Can you work these out from the model? Positions are in its coordinate system, mm. Face numbers are marked on the shaded views. A direction names the side the tool comes from. Round coordinates to 2 decimals unless told otherwise and drop trailing zeros. Loops run counter-clockwise (first coordinate to the right, second up) from the corner with the lowest first, then second, coordinate; pieces in that order, holes last. Notation, with made-up numbers: (67.25, 79) - (116.25, 79) arc R23 ccw to (116.25, 115) - close; hole circle Ø1 at (41, -30.5). An arc over 180 degrees is marked (long way). Answer as CSV lines item,"result".
```python
from build123d import *

# Parameters (mm, degrees)
SKETCH1_W           = 50
SKETCH1_H           = 40
BOSS_EXTRUDE1_DEPTH = 50
SKETCH2_W           = 44
SKETCH2_H           = 44
CUT_EXTRUDE1_DEPTH  = 50
SKETCH3_R           = 1.7
CUT_EXTRUDE3_DEPTH  = 78.691698398
SKETCH5_R           = 9
CUT_EXTRUDE4_DEPTH  = 2
SKETCH6_R           = 3
CUT_EXTRUDE5_DEPTH  = 79.841613378
SKETCH7_R           = 1.7
CUT_EXTRUDE6_DEPTH  = 78.691698398


with BuildPart() as part:
    # Sketch1 → Boss-Extrude1 (new body)
    with BuildSketch(Plane(origin=(0, 0, 0), x_dir=(1, 0, 0), z_dir=(0, 1, 0))):
        with Locations((25, 20)):
            Rectangle(SKETCH1_W, SKETCH1_H)
    extrude(amount=BOSS_EXTRUDE1_DEPTH)

    # Sketch2 → Cut-Extrude1 (cut)
    with BuildSketch(Plane.XY):
        with Locations((22, 28)):
            Rectangle(SKETCH2_W, SKETCH2_H)
    extrude(amount=-CUT_EXTRUDE1_DEPTH, mode=Mode.SUBTRACT)

    # Sketch3 → Cut-Extrude3 (cut, through all)
    with BuildSketch(Plane.ZY.offset(-44)):
        with Locations(Location((-30, 40, 0), (0, 0, 270))):
            Circle(SKETCH3_R)
        with Locations(Location((-10, 40, 0), (0, 0, 270))):
            Circle(SKETCH3_R)
        with Locations(Location((-10, 16, 0), (0, 0, 270))):
            Circle(SKETCH3_R)
        with Locations(Location((-30, 16, 0), (0, 0, 270))):
            Circle(SKETCH3_R)
    extrude(amount=-CUT_EXTRUDE3_DEPTH, mode=Mode.SUBTRACT)

    # Sketch5 → Cut-Extrude4 (cut)
    with BuildSketch(Plane(origin=(0, 6, 0), x_dir=(1, 0, 0), z_dir=(0, 1, 0))):
        with Locations(Location((23, 20, 0), (0, 0, 270))):
            Circle(SKETCH5_R)
    extrude(amount=-CUT_EXTRUDE4_DEPTH, mode=Mode.SUBTRACT)

    # Sketch6 → Cut-Extrude5 (cut, through all)
    with BuildSketch(Plane(origin=(0, 4, 0), x_dir=(1, 0, 0), z_dir=(0, 1, 0))):
        with Locations(Location((23, 20, 0), (0, 0, 270))):
            Circle(SKETCH6_R)
    extrude(amount=-CUT_EXTRUDE5_DEPTH, mode=Mode.SUBTRACT)

    # Sketch7 → Cut-Extrude6 (cut, through all)
    with BuildSketch(Plane(origin=(0, 6, 0), x_dir=(1, 0, 0), z_dir=(0, 1, 0))):
        with Locations(Location((12, 20, 0), (0, 0, 270))):
            Circle(SKETCH7_R)
        with Locations(Location((23, 31, 0), (0, 0, 270))):
            Circle(SKETCH7_R)
        with Locations(Location((34, 20, 0), (0, 0, 270))):
            Circle(SKETCH7_R)
        with Locations(Location((23, 9, 0), (0, 0, 270))):
            Circle(SKETCH7_R)
    extrude(amount=-CUT_EXTRUDE6_DEPTH, mode=Mode.SUBTRACT)


solid = part.part
```
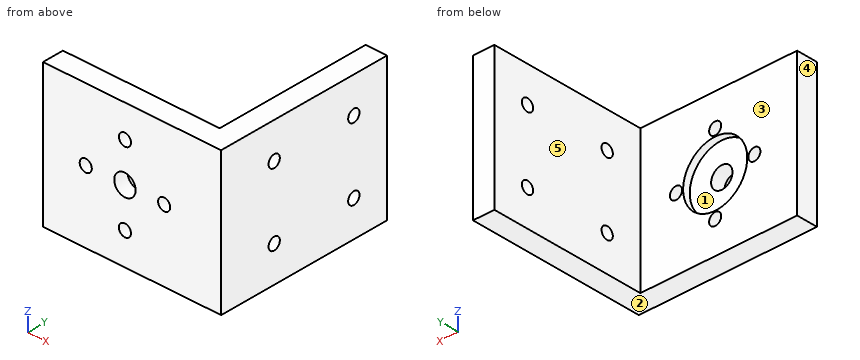
Q1. I'm going to push flat-ended pins straight in: pin 1 Ø14.5 at (x, z) = (19.5, -19) entering from +Y; pin 2 Ø2.5 at (y, z) = (16, -10) entering from -X; pin 3 Ø20 at (y, z) = (25.5, -21.5) entering from -X; pin 4 Ø1.5 at (x, z) = (20.5, -19.5) entering from +Y. Where does each tip first touch, or does it pass through?
Checks:
pin 1,"y = 6"
pin 2,"through"
pin 3,"x = 44"
pin 4,"y = 4"
Q2. Imagine slicing it at A-A (x = 34). Write out the boundary of the cut face in (y, z), then the cut area to 3 significant figures.
Checks:
outline,"(0, -40) - (6, -40) - (6, -21.7) - (0, -21.7) - close; (0, -18.3) - (6, -18.3) - (6, 0) - (0, 0) - close"
area,"220 mm²"
Q3. If I drill on line 1 along X through (y, z) = (2, -20); line 2 along X through (y, z) = (5.2, -20); line 3 along Z through (x, y) = (46.7, 16), over which ranges is the centre line in solid material (lowest first)? Write a range as [from, to].
Checks:
line 1,"[0, 10.3], [13.7, 20], [26, 32.3], [35.7, 50]"
line 2,"[0, 10.3], [13.7, 14], [32, 32.3], [35.7, 50]"
line 3,"[-40, -31.7], [-28.3, -11.7], [-8.3, 0]"
Q4. Imagine slicing it at D-D (z = -31). Write out the boundary of the cut face in (x, y), then the cut area to 3 significant figures.
Checks:
outline,"(0, 0) - (21.3, 0) - (21.3, 6) - (0, 6) - close; (24.7, 0) - (50, 0) - (50, 14.63) - (44, 14.63) - (44, 6) - (24.7, 6) - close; (44, 17.37) - (50, 17.37) - (50, 38.63) - (44, 38.63) - close; (44, 41.37) - (50, 41.37) - (50, 50) - (44, 50) - close"
area,"511 mm²"
Q5. On a 3-axis mill with a long thin cutter (end or side, diameter ignored), from which of +Z, -Z, +X, -X, +Y, -Y can I reach the whole of each face in a straight line? I mean the marked faces 4 and 5. Say none if no direction works.
Checks:
face 4,"+Z, -Z, -X, +Y, -Y"
face 5,"+Z, -Z, -X, +Y"
Q6. Imagine slicing it at C-C (x = 22). Write out the boundary of the cut face in (y, z).
Checks:
outline,"(0, -40) - (6, -40) - (6, -32.37) - (0, -32.37) - close; (0, -29.63) - (6, -29.63) - (6, -28.94) - (4, -28.94) - (4, -22.83) - (0, -22.83) - close; (0, -17.17) - (4, -17.17) - (4, -11.06) - (6, -11.06) - (6, -10.37) - (0, -10.37) - close; (0, -7.63) - (6, -7.63) - (6, 0) - (0, 0) - close"
Q7. We'd pull the mould along Z, two halves only. Please class the marked faces 1, 2 and 3: pulls with the +Z half, pulls with the -Z half, needs draft (parallel to the pull), parting line crosses it, or undercut.
Checks:
face 1,"undercut"
face 2,"pulls with the -Z half"
face 3,"needs draft"
Q8. Imagine slicing it at B-B (z = -5.5). Write out the boundary of the cut face in (x, y), then the cut area to 3 significant figures.
Checks:
outline,"(0, 0) - (50, 0) - (50, 50) - (44, 50) - (44, 6) - (0, 6) - close"
area,"564 mm²"
